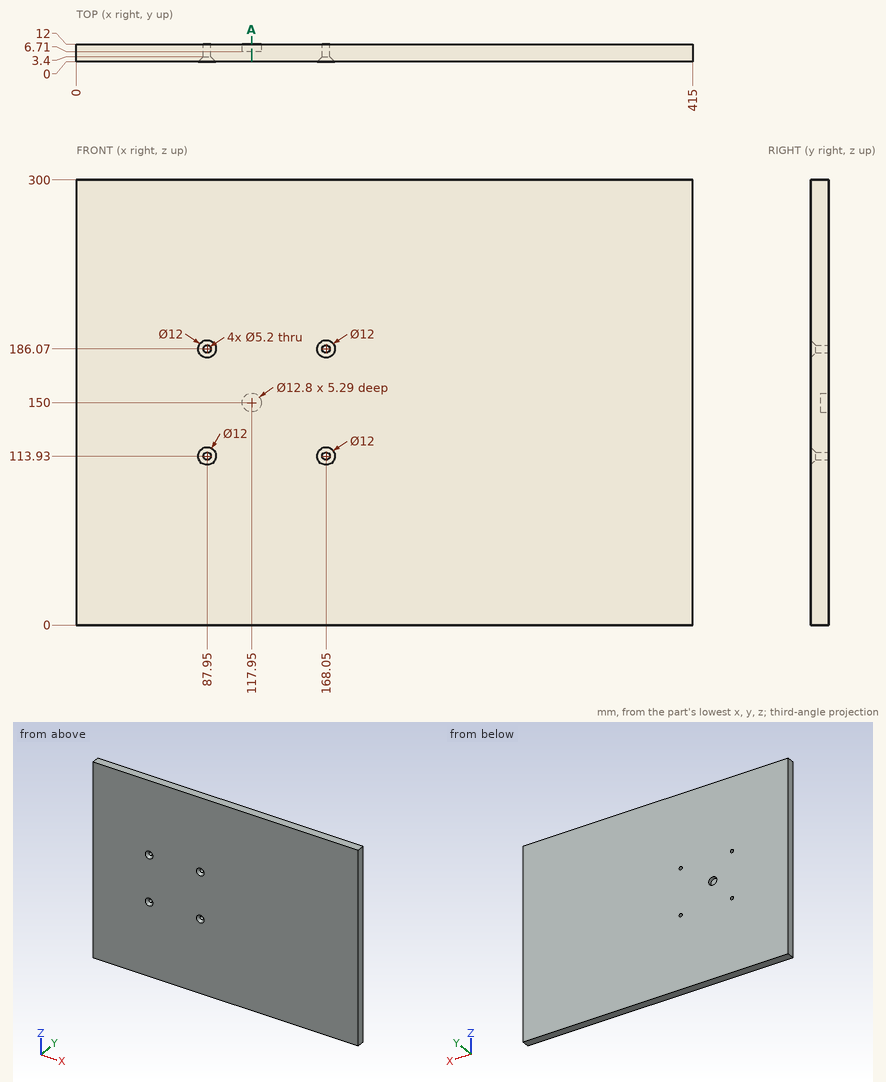
Design review of the part shown in the three views and the two pictorial views. Dimensions are in mm from the part's minimum x, y and z. Round coordinates to 2 decimals unless told otherwise and drop trailing zeros. Loops run counter-clockwise (first coordinate to the right, second up) from the corner with the lowest first, then second, coordinate; pieces in that order, holes last. Notation, with made-up numbers: M -11,9.25 L 34,9.25 A22 ccw 34,44.25 Z; hole C 50.5,5 d1. An arc over 180 degrees is marked long. Answer as a JSON object with one key per item and string values.
Item 1: We need section A-A, the plane x = 117.95. State the section outline as (y, z) points.
Check sheet entries:
{"outline": "M 0,0 L 12,0 L 12,143.6 L 6.71,143.6 L 6.71,156.4 L 12,156.4 L 12,300 L 0,300 Z"}
Item 2: For line 1 along X through (y, z) = (9, 113.93); line 2 along Z through (x, y) = (168.05, 5.5); line 3 along Z through (x, y) = (117.95, 9.1), list the stretches that pass through material, from the lowest coordinate up.
Check sheet entries:
{"line 1": "0 to 85.35, 90.55 to 165.45, 170.65 to 415", "line 2": "0 to 111.33, 116.53 to 183.47, 188.67 to 300", "line 3": "0 to 143.6, 156.4 to 300"}
Item 3: Clearance check with flat-ended pins moving along their axes: P1, Ø4, axis at x = 87.95, z = 113.93, coming from the -Y side; P2, Ø4, axis at x = 119.5, z = 150.5, coming from the +Y side. State where each tip first meets the part, or that it passes through.
Check sheet entries:
{"P1": "through", "P2": "y = 6.71"}
